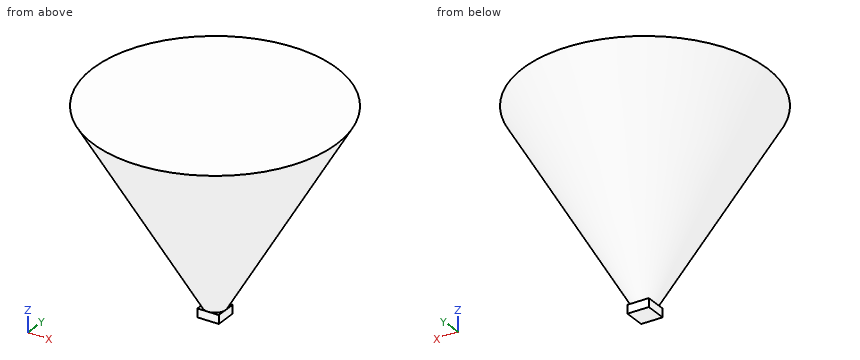
Autodesk Inventor part; units mm, degrees
ref_plane "YZ Plane" through (0, 0, 0) normal (1, 0, 0) x (0, 1, 0)
ref_plane "XZ Plane" through (0, 0, 0) normal (0, 1, 0) x (-1, 0, 0)
ref_plane "XY Plane" through (0, 0, 0) normal (0, 0, 1) x (1, 0, 0)
sketch "Sketch1" plane through (0, 0, 0) normal (0, 0, 1) x (1, 0, 0)
  line L0 (-2.5, 2.5) -> (2.5, 2.5)
  line L1 (2.5, 2.5) -> (2.5, -2.5)
  line L2 (2.5, -2.5) -> (-2.5, -2.5)
  line L3 (-2.5, -2.5) -> (-2.5, 2.5)
  line L4 (-2.5, 2.5) -> (2.5, -2.5) construction
  line L5 (2.5, 2.5) -> (-2.5, -2.5) construction
  circle A0 centre (0, 0) radius 2.25
  dimension "d0" = 5
  dimension "d1" = 5
  dimension "d2" = 4.5
extrude "Extrusion1" add sketch "Sketch1" along normal blind 2 contours L0 L1 L2 L3 | A0
sketch "Sketch2" plane through (-2.5, -2.5, 0) normal (0, -1, 0) x (1, 0, 0)
  line L0 (5, 0) -> (0, 0)
  line L1 (5, 0) -> (5, 2)
  line L2 (0, 2) -> (5, 2)
  line L3 (0, 0) -> (0, 2)
  line L4 (5, 2) -> (0, 2)
  line L5 (0, 2) -> (-25.9808, 47)
  line L6 (-25.9808, 47) -> (30.9808, 47)
  line L7 (5, 2) -> (30.9808, 47)
  point P0 (2.5, 0)
  dimension "d5" = 120
  dimension "d6" = 120
  dimension "d7" = 45
  dimension "d9" = 56.9615
sketch "Sketch3" plane through (0, 0, 2) normal (0, 0, 1) x (1, 0, 0)
  circle A0 centre (0, 0) radius 2.5
ref_plane "Work Plane1" through (0, 0, 47) normal (0, 0, 1) x (1, 0, 0)
sketch "Sketch4" plane through (0, 0, 47) normal (0, 0, 1) x (1, 0, 0)
  circle A0 centre (0, 0) radius 28.5
  point P0 (28.4808, -2.5)
  dimension "d10" = 57
loft "Loft1" add profiles "Sketch3", "Sketch4"
equation "\"d6\" = d5"
properties part number "led 5050"
Check sheet for the modelled part. Datum: model origin and axes. Units: mm. Give positions to 0.01 mm unless a question says otherwise; leave off trailing zeros. Loops run counter-clockwise (first coordinate to the right, second up) from the corner with the lowest first, then second, coordinate; pieces in that order, holes last. Notation, with made-up numbers: M 12,0.25 L 57,0.25 A10 cw 57,12.25 Z; hole C -9,64 d4. An arc over 180 degrees is marked long. Return JSON: item names as keys, results as strings. Group by question number.
1. Go/stop test with flat-tipped pins: pin 1 (1.6 mm diameter, centred on x = 1, z = 0.5, fed in from -Y); pin 2 (1 mm diameter, centred on x = 1.5, y = -13.5, fed in from -Z); pin 3 (2 mm diameter, centred on y = 1, z = 0.5, fed in from -X). Record where each tip stops, or that it passes through.
2. Cross-section at B-B on z = 24. Record the boundary of the cut face in (x, y).
3. Thickness scan on L1, parallel to Y at x = 10.5, z = 26.5; L2, parallel to Y at x = -4.5, z = 31.5; L3, parallel to X at y = -14, z = 34. Record the ranges inside material, lowest first.
4. Cross-section at A-A on z = 15.5. Record the boundary of the cut face in (x, y), plus the area to 3 significant figures.
Return value:
{
 "1": {"pin 1": "y = -2.5", "pin 2": "z = 20.32", "pin 3": "x = -2.5"},
 "2": {"outline": "C 0,0 d30.42"},
 "3": {"L1": "-12.93 to 12.93", "L2": "-19.02 to 19.02", "L3": "-15.64 to 15.64"},
 "4": {"outline": "C 0,0 d20.6", "area": "333 mm^2"}
}
